Could you check a few things on this model? Use its own coordinates, in mm. Round coordinates to 2 decimals unless told otherwise and drop trailing zeros. Order: outer loops, then holes, each group sorted by start corner. A loop starts at its lowest first (then second) coordinate and runs counter-clockwise, first axis right, second up. Notation, with made-up numbers: (81.5, 24) - (123.5, 24) arc R19 cw to (123.5, 43) - close; hole circle Ø5 at (-18, 75.25). An arc over 180 degrees is marked (long way). Use one line per item in the form item = value.
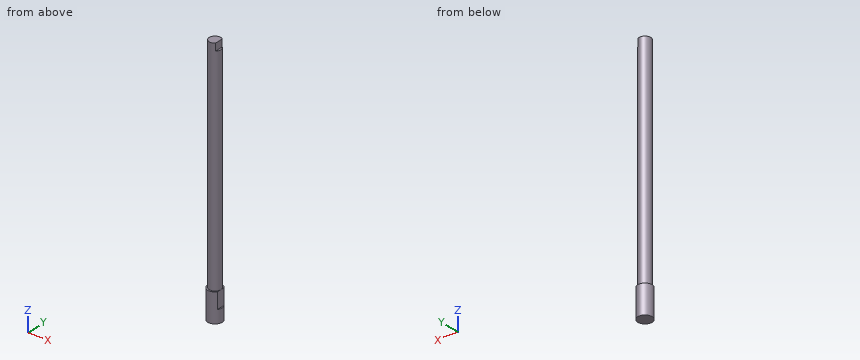
Solid Edge part; units mm, degrees
sketch "Sketch1" plane through (0, 0, 0) normal (0, 0, 1) x (1, 0, 0)
  circle A0 centre (0, 0) radius 5
extrude "Protrusion1" add sketch "Sketch1" along normal blind 20
sketch "Sketch2" plane through (0, 0, 20) normal (0, 0, 1) x (1, 0, 0)
  circle A0 centre (0, 0) radius 4
extrude "ExtrudedProtrusion_2" add sketch "Sketch2" along normal blind 155
sketch "Sketch3" plane through (0, 0, 20) normal (0, 0, 1) x (0, -1, 0)
  line L0 (-3.8216, 6.2347) -> (3.8216, 6.2347)
  line L1 (3.8216, 6.2347) -> (3.8216, 4)
  line L2 (3.8216, 4) -> (0, 4)
  line L3 (0, 4) -> (-3.8216, 4)
  line L4 (-3.8216, 4) -> (-3.8216, 6.2347)
extrude "ExtrudedCutout_1" cut sketch "Sketch3" against normal blind 11.0575
sketch "Sketch4" plane through (0, 0, 175) normal (0, 0, 1) x (0, -1, 0)
  line L0 (-3.2306, 4) -> (4.2507, 4)
  line L1 (4.2507, 4) -> (4.2507, 2.6458)
  line L2 (4.2507, 2.6458) -> (0, 2.6458)
  line L3 (0, 2.6458) -> (-3.2306, 2.6458)
  line L4 (-3.2306, 2.6458) -> (-3.2306, 4)
extrude "ExtrudedCutout_2" cut sketch "Sketch4" against normal blind 5
Item 1: Imagine slicing it at A-A on x = 0. Please give me the cut outline in (y, z).
Found:
outline = (-5, 0) - (5, 0) - (5, 20) - (4, 20) - (4, 175) - (-4, 175) - (-4, 20) - (-5, 20) - close
Item 2: I need wall thicknesses on L1, parallel to Y at x = 0.25, z = 87; L2, parallel to Z at x = 0, y = 4.5; L3, parallel to X at y = 4, z = 12. Which ranges of each line are inside material? Lowest first, please.
Found:
L1 = -3.99 to 3.99
L2 = 0 to 20
L3 = -3 to 3
Item 3: Will these pins go through, and if not, where does the flat tip stop? P1, Ø6, axis at y = -3.5, z = 67.5, coming from the +X side; P2, Ø3, axis at y = -0.5, z = 120.5, coming from the -X side; P3, Ø0.5, axis at x = 4.5, y = 0, coming from the +Z side.
Found:
P1 = 3.97
P2 = -4
P3 = 8.94
Item 4: Imagine slicing it at B-B on z = 29.5. Please give me the cut outline in (x, y), plus the area to 3 significant figures.
Found:
outline = circle Ø8 at (0, 0)
area = 50.3 mm2
